```python
from build123d import *

# Parameters (mm, degrees)
F3_DEPTH = 12.5
F2_R     = 6.477
F4_DEPTH = 7.62
F5_R     = 2.54
F6_DEPTH = 25.4


with BuildPart() as f1:
    # F0 (on Front) → F1 (revolve)
    with BuildSketch(Plane.XZ):
        Polygon((-25.4, 0), (0, 0), (0, 16), (-6.35, 16), (-6.35, 17.5), (-8.89, 17.5), (-8.89, 19), (-11.43, 19), (-11.43, 20.5), (-13.97, 20.5), (-13.97, 22), (-16.51, 22), (-16.51, 23.5), (-19.05, 23.5), (-19.05, 25), (-21.59, 25), (-23.8, 20), (-23.8, 12.5), (-25.4, 12.5), align=None)
    revolve(axis=Axis((0, 0, 8), (0, 0, -1)))

    # F2 (on face) → F3 (join)
    with BuildSketch(Plane(origin=(0, 0, 0), x_dir=(1, 0, 0), z_dir=(0, 0, -1))):
        with BuildLine():
            ThreePointArc((-25.3803149606, -0.9998062308), (-25.4, 0), (-25.3803149606, 0.9998062308))
            ThreePointArc((-25.3803149606, 0.9998062308), (-26.4, 0), (-25.3803149606, -0.9998062308))
        make_face()
        with BuildLine():
            ThreePointArc((-21.4800943965, 13.5560150751), (-21.9970452561, 12.7), (-22.4799006274, 11.8242998855))
            ThreePointArc((-22.4799006274, 11.8242998855), (-21.4885451928, 11.8389380477), (-20.9970452561, 12.7))
            ThreePointArc((-20.9970452561, 12.7), (-21.1261403074, 13.1914514932), (-21.4800943965, 13.5560150751))
        make_face()
        with BuildLine():
            ThreePointArc((-21.4800943965, 13.5560150751), (-22.8630706599, 13.2), (-22.4799006274, 11.8242998855))
            ThreePointArc((-22.4799006274, 11.8242998855), (-21.9970452561, 12.7), (-21.4800943965, 13.5560150751))
        make_face()
        with BuildLine():
            ThreePointArc((-21.4800943965, -13.5560150751), (-21.9970452561, -12.7), (-22.4799006274, -11.8242998855))
            ThreePointArc((-22.4799006274, -11.8242998855), (-22.8630706599, -13.2), (-21.4800943965, -13.5560150751))
        make_face()
        with BuildLine():
            ThreePointArc((-11.8242998855, 22.4799006274), (-12.7, 21.9970452561), (-13.5560150751, 21.4800943965))
            ThreePointArc((-13.5560150751, 21.4800943965), (-12.4316858884, 21.0337137776), (-11.7, 21.9970452561))
            ThreePointArc((-11.7, 21.9970452561), (-11.7315734115, 22.2463441586), (-11.8242998855, 22.4799006274))
        make_face()
        with BuildLine():
            ThreePointArc((-11.8242998855, 22.4799006274), (-13.2, 22.8630706599), (-13.5560150751, 21.4800943965))
            ThreePointArc((-13.5560150751, 21.4800943965), (-12.7, 21.9970452561), (-11.8242998855, 22.4799006274))
        make_face()
        with BuildLine():
            ThreePointArc((-11.8242998855, -22.4799006274), (-12.7, -21.9970452561), (-13.5560150751, -21.4800943965))
            ThreePointArc((-13.5560150751, -21.4800943965), (-13.2, -22.8630706599), (-11.8242998855, -22.4799006274))
        make_face()
        with BuildLine():
            ThreePointArc((0.9998062308, 25.3803149606), (0, 25.4), (-0.9998062308, 25.3803149606))
            ThreePointArc((-0.9998062308, 25.3803149606), (0, 24.4), (0.9998062308, 25.3803149606))
        make_face()
        with BuildLine():
            ThreePointArc((1, 25.4), (-0.0098429965, 26.3999515565), (-0.9998062308, 25.3803149606))
            ThreePointArc((-0.9998062308, 25.3803149606), (0, 25.4), (0.9998062308, 25.3803149606))
            ThreePointArc((0.9998062308, 25.3803149606), (0.9999515565, 25.3901570035), (1, 25.4))
        make_face()
        with BuildLine():
            ThreePointArc((0.9998062308, -25.3803149606), (0, -25.4), (-0.9998062308, -25.3803149606))
            ThreePointArc((-0.9998062308, -25.3803149606), (-0.0098429965, -26.3999515565), (1, -25.4))
            ThreePointArc((1, -25.4), (0.9999515565, -25.3901570035), (0.9998062308, -25.3803149606))
        make_face()
        with BuildLine():
            ThreePointArc((13.5560150751, 21.4800943965), (12.7, 21.9970452561), (11.8242998855, 22.4799006274))
            ThreePointArc((11.8242998855, 22.4799006274), (12.2, 21.1310198523), (13.5560150751, 21.4800943965))
        make_face()
        with BuildLine():
            ThreePointArc((13.7, 21.9970452561), (12.9492989025, 22.9654718446), (11.8242998855, 22.4799006274))
            ThreePointArc((11.8242998855, 22.4799006274), (12.7, 21.9970452561), (13.5560150751, 21.4800943965))
            ThreePointArc((13.5560150751, 21.4800943965), (13.6633314785, 21.7287311446), (13.7, 21.9970452561))
        make_face()
        with BuildLine():
            ThreePointArc((13.5560150751, -21.4800943965), (12.7, -21.9970452561), (11.8242998855, -22.4799006274))
            ThreePointArc((11.8242998855, -22.4799006274), (12.9492989025, -22.9654718446), (13.7, -21.9970452561))
            ThreePointArc((13.7, -21.9970452561), (13.6633314785, -21.7287311446), (13.5560150751, -21.4800943965))
        make_face()
        with BuildLine():
            ThreePointArc((22.4799006274, 11.8242998855), (21.9970452561, 12.7), (21.4800943965, 13.5560150751))
            ThreePointArc((21.4800943965, 13.5560150751), (21.1310198523, 12.2), (22.4799006274, 11.8242998855))
        make_face()
        with BuildLine():
            ThreePointArc((22.9970452561, 12.7), (22.4884967494, 13.5709049488), (21.4800943965, 13.5560150751))
            ThreePointArc((21.4800943965, 13.5560150751), (21.9970452561, 12.7), (22.4799006274, 11.8242998855))
            ThreePointArc((22.4799006274, 11.8242998855), (22.8581072084, 12.1914999367), (22.9970452561, 12.7))
        make_face()
        with BuildLine():
            ThreePointArc((22.4799006274, -11.8242998855), (21.9970452561, -12.7), (21.4800943965, -13.5560150751))
            ThreePointArc((21.4800943965, -13.5560150751), (22.4884967494, -13.5709049488), (22.9970452561, -12.7))
            ThreePointArc((22.9970452561, -12.7), (22.8581072084, -12.1914999367), (22.4799006274, -11.8242998855))
        make_face()
        with BuildLine():
            ThreePointArc((26.4, 0), (26.1001124769, 0.7140325761), (25.3803149606, 0.9998062308))
            ThreePointArc((25.3803149606, 0.9998062308), (25.3950782633, 0.5), (25.4, 0))
            ThreePointArc((25.4, 0), (25.3950782633, -0.5), (25.3803149606, -0.9998062308))
            ThreePointArc((25.3803149606, -0.9998062308), (26.1001124769, -0.7140325761), (26.4, 0))
        make_face()
    extrude(amount=-F3_DEPTH)

    # F2 (on face) → F4 (cut)
    with BuildSketch(Plane(origin=(0, 0, 0), x_dir=(1, 0, 0), z_dir=(0, 0, -1))):
        Circle(F2_R)
    extrude(amount=-F4_DEPTH, mode=Mode.SUBTRACT)

    # F5 (on face) → F6 (cut)
    with BuildSketch(Plane.XY.offset(16)):
        Circle(F5_R)
    extrude(amount=-F6_DEPTH, mode=Mode.SUBTRACT)


solid = f1.part
```
Geometry check sheet. Reference: the model listing, model coordinates, mm. A direction names the side the tool comes from. Coordinates: 2 decimals unless noted, no trailing zeros. Order: outer loops, then holes, each group sorted by start corner. A loop starts at its lowest first (then second) coordinate and runs counter-clockwise, first axis right, second up. Notation, with made-up numbers: (40.5, -2.5) - (89.5, -2.5) arc R23 cw to (89.5, 26.5) - close; hole circle Ø5 at (-12, -13). An arc over 180 degrees is marked (long way). Answer as a JSON object with one key per item and string values. Group by question number.
Item 1: Tool access check on faces 1 (the face through (4, -6, 17.5)), 2 (the face through (-13.22, 22.85, 6.16)). Record the directions out of +Z, -Z, +X, -X, +Y, -Y that give a thin tool (end or side, any length) a straight path to the whole face; none if there is none.
Item 2: Depth check by flat-ended pin: pin 1 Ø14 at (x, y) = (1, 1) entering from -Z; pin 2 Ø10 at (y, z) = (14, 16.5) entering from +X; pin 3 Ø8 at (x, z) = (-5.5, 12) entering from +Y; pin 4 Ø5 at (x, z) = (14, 18) entering from +Y. Enter the tip coordinate at first touch or a pass-through.
Item 3: Scan lines: probe 1 along Y at (x, z) = (0, 18.7); probe 2 along Y at (x, z) = (0, 22.75); probe 3 along Z at (x, y) = (-11.5, -2.5). Record each from-to range of solid material in increasing order.
Item 4: Draft check along Y on faces 3 (the face through (7.9, -17.5, 25)), 4 (the face through (1.38, -6.2, 16.76)), 5 (the face through (-6.7, 24.5, 6.2)), 6 (the face through (-20.725, 6.527, 24.687)). Enter one of: +Y half, -Y half, draft (parallel to the pull), parting line (faces both ways), or undercut.
Item 5: Sectioned sample at A-A, the plane z = 5.5. Record the cut outline in (x, y).
Resolved:
{
 "1": {"face 1": "+Z", "face 2": "+Z, -Z"},
 "2": {"pin 1": "z = 0", "pin 2": "x = 23", "pin 3": "y = 25.36", "pin 4": "y = 20.84"},
 "3": {"probe 1": "-23.8 to -8.89, 8.89 to 23.8", "probe 2": "-22.58 to -16.51, 16.51 to 22.58", "probe 3": "0 to 20.5"},
 "4": {"face 3": "draft", "face 4": "undercut", "face 5": "+Y half", "face 6": "parting line"},
 "5": {"outline": "(-25.38, -1) arc R25.4 ccw to (-22.48, -11.82) arc R1 ccw (long way) to (-21.48, -13.56) arc R25.4 ccw to (-13.56, -21.48) arc R1 ccw (long way) to (-11.82, -22.48) arc R25.4 ccw to (-1, -25.38) arc R1 ccw (long way) to (1, -25.38) arc R25.4 ccw to (11.82, -22.48) arc R1 ccw (long way) to (13.56, -21.48) arc R25.4 ccw to (21.48, -13.56) arc R1 ccw (long way) to (22.48, -11.82) arc R25.4 ccw to (25.38, -1) arc R1 ccw (long way) to (25.38, 1) arc R25.4 ccw to (22.48, 11.82) arc R1 ccw (long way) to (21.48, 13.56) arc R25.4 ccw to (13.56, 21.48) arc R1 ccw (long way) to (11.82, 22.48) arc R25.4 ccw to (1, 25.38) arc R1 ccw (long way) to (-1, 25.38) arc R25.4 ccw to (-11.82, 22.48) arc R1 ccw (long way) to (-13.56, 21.48) arc R25.4 ccw to (-21.48, 13.56) arc R1 ccw (long way) to (-22.48, 11.82) arc R25.4 ccw to (-25.38, 1) arc R1 ccw (long way) to start; hole circle Ø12.95 at (0, 0)"}
}
